from build123d import *

# Parameters (mm, degrees)
SKETCH1_R           = 24
SKETCH1_R_2         = 1.5
BOSS_EXTRUDE1_DEPTH = 0.8


with BuildPart() as part:
    # Sketch1 → Boss-Extrude1 (new, symmetric)
    with BuildSketch(Plane(origin=(0, 0, 0), x_dir=(1, 0, 0), z_dir=(0, 1, 0))):
        with Locations(Location((0, 0, 0), (0, 0, 270))):
            Circle(SKETCH1_R)
        with Locations(Location((-19.75, 0, 0), (0, 0, 270))):
            Circle(SKETCH1_R_2, mode=Mode.SUBTRACT)
        with Locations(Location((0, -19.75, 0), (0, 0, 270))):
            Circle(SKETCH1_R_2, mode=Mode.SUBTRACT)
        with Locations(Location((19.75, 0, 0), (0, 0, 270))):
            Circle(SKETCH1_R_2, mode=Mode.SUBTRACT)
        with Locations(Location((0, 19.75, 0), (0, 0, 270))):
            Circle(SKETCH1_R_2, mode=Mode.SUBTRACT)
    extrude(amount=BOSS_EXTRUDE1_DEPTH, both=True)


solid = part.part
Can you work these out from the model? Positions are in its coordinate system, mm. Coordinates: 2 decimals unless noted, no trailing zeros. Order: outer loops, then holes, each group sorted by start corner. A loop starts at its lowest first (then second) coordinate and runs counter-clockwise, first axis right, second up. Notation, with made-up numbers: (-26.75, 42.25) - (-1.75, 42.25) arc R6 cw to (-1.75, 53.25) - close; hole circle Ø11 at (10, 85). An arc over 180 degrees is marked (long way). Answer as a JSON object with one key per item and string values. Group by question number.
Q1. Imagine slicing it at D-D (x = 19.75). Please give me the cut outline in (y, z).
Q2. We'd pull the mould along X, two halves only. Please class faces 1 (the face through (-18.485, -0.011, 0.806)), 2 (the face through (7.21, 0.01, 22.89)), 3 (the face through (0, 0.8, 0)): +X half, -X half, draft (parallel to the pull), parting line (faces both ways), or undercut.
Q3. I need wall thicknesses on line 1 (X direction, y = 0.4, z = 0); line 2 (Z direction, x = 18.5, y = -0.3); line 3 (X direction, y = 0, z = 19.75). Which ranges of each line are inside material? Lowest first, please. Write a range as from..to.
Q4. Imagine slicing it at B-B (y = -0.3). Please give me the cut outline in (x, z), and give its area (3 significant figures).
Q5. Imagine slicing it at C-C (z = 19.75). Please give me the cut outline in (x, y), and give its area (3 significant figures).
Q6. Will these pins go through, and if not, where does the flat tip stop? P1, Ø2.5, axis at x = 0, z = 19.75, coming from the -Y side; P2, Ø3.5, axis at x = 19.75, z = 0, coming from the -Y side.
Q7. Imagine slicing it at A-A (z = 0). Please give me the cut outline in (x, y), and give its area (3 significant figures).
Determined:
{
 "1": {"outline": "(-0.8, -13.64) - (0.8, -13.64) - (0.8, -1.5) - (-0.8, -1.5) - close; (-0.8, 1.5) - (0.8, 1.5) - (0.8, 13.64) - (-0.8, 13.64) - close"},
 "2": {"face 1": "undercut", "face 2": "parting line", "face 3": "draft"},
 "3": {"line 1": "x = -24..-21.25, -18.25..18.25, 21.25..24", "line 2": "z = -15.29..-0.83, 0.83..15.29", "line 3": "x = -13.64..-1.5, 1.5..13.64"},
 "4": {"outline": "circle Ø48 at (0, 0); hole circle Ø3 at (-19.75, 0); hole circle Ø3 at (0, -19.75); hole circle Ø3 at (0, 19.75); hole circle Ø3 at (19.75, 0)", "area": "1,780 mm2"},
 "5": {"outline": "(-13.64, -0.8) - (-1.5, -0.8) - (-1.5, 0.8) - (-13.64, 0.8) - close; (1.5, -0.8) - (13.64, -0.8) - (13.64, 0.8) - (1.5, 0.8) - close", "area": "38.8 mm2"},
 "6": {"P1": "passes through", "P2": "stops at y = -0.8"},
 "7": {"outline": "(-24, -0.8) - (-21.25, -0.8) - (-21.25, 0.8) - (-24, 0.8) - close; (-18.25, -0.8) - (18.25, -0.8) - (18.25, 0.8) - (-18.25, 0.8) - close; (21.25, -0.8) - (24, -0.8) - (24, 0.8) - (21.25, 0.8) - close", "area": "67.2 mm2"}
}
